```python
from build123d import *

# Parameters (mm, degrees)
BOSS_EXTRUDE1_DEPTH      = 60
BOSS_EXTRUDE1_DEPTH_BACK = 20
SKETCH2_R                = 1.7
CUT_EXTRUDE1_DEPTH       = 10
BOSS_EXTRUDE2_START      = 24
BOSS_EXTRUDE2_DEPTH      = 24
CUT_EXTRUDE2_START       = -10
SKETCH4_R                = 1.7
CUT_EXTRUDE2_DEPTH       = 10


with BuildPart() as part:
    # Sketch1 → Boss-Extrude1 (new, two sides: drawn at the far end of the back side and taken through both)
    with BuildSketch(Plane(origin=(190.645148, 0, 0), x_dir=(0, 0, -1), z_dir=(1, 0, 0)).offset(-BOSS_EXTRUDE1_DEPTH_BACK)):
        with BuildLine():
            Line((-240.970904961, 189.163538159), (-246.970904961, 189.163538159))
            Line((-246.970904961, 189.163538159), (-246.970904961, 173.663538158))
            Line((-246.970904961, 173.663538158), (-240.970904961, 173.663538158))
            Line((-240.970904961, 173.663538158), (-240.970904961, 179.413538158))
            Line((-240.970904961, 179.413538158), (-241.970904961, 179.413538158))
            ThreePointArc((-241.970904961, 179.413538158), (-243.970904961, 181.413538158), (-241.970904961, 183.413538158))
            Line((-241.970904961, 183.413538158), (-240.970904961, 183.413538158))
            Line((-240.970904961, 183.413538158), (-240.970904961, 189.163538159))
        make_face()
    extrude(amount=BOSS_EXTRUDE1_DEPTH + BOSS_EXTRUDE1_DEPTH_BACK)

    # Sketch2 → Cut-Extrude1 (cut)
    with BuildSketch(Plane.XY.offset(246.970904961)):
        with Locations((246.645148, 186.288538158)):
            Circle(SKETCH2_R)
        with Locations((222.645148, 186.288538158)):
            Circle(SKETCH2_R)
        with Locations((198.645148, 186.288538158)):
            Circle(SKETCH2_R)
        with Locations((174.645148, 186.288538158)):
            Circle(SKETCH2_R)
        with Locations((246.645148, 176.593153442)):
            Circle(SKETCH2_R)
        with Locations((222.645148, 176.593153442)):
            Circle(SKETCH2_R)
        with Locations((198.645148, 176.593153442)):
            Circle(SKETCH2_R)
        with Locations((174.645148, 176.593153442)):
            Circle(SKETCH2_R)
    extrude(amount=-CUT_EXTRUDE1_DEPTH, mode=Mode.SUBTRACT)

    # Sketch3 → Boss-Extrude2 (add)
    with BuildSketch(Plane.ZY.offset(-170.645148).offset(BOSS_EXTRUDE2_START)):
        with BuildLine():
            Line((241.970904961, 179.413538158), (240.970904961, 179.413538158))
            Line((240.970904961, 179.413538158), (240.970904961, 173.663538158))
            Line((240.970904961, 173.663538158), (246.970904961, 173.663538158))
            Line((246.970904961, 173.663538158), (246.970904961, 189.163538159))
            Line((246.970904961, 189.163538159), (240.970904961, 189.163538159))
            Line((240.970904961, 189.163538159), (240.970904961, 183.413538158))
            Line((240.970904961, 183.413538158), (241.970904961, 183.413538158))
            ThreePointArc((241.970904961, 183.413538158), (243.970904961, 181.413538158), (241.970904961, 179.413538158))
        make_face()
    extrude(amount=-BOSS_EXTRUDE2_DEPTH)

    # Sketch4 → Cut-Extrude2 (cut)
    with BuildSketch(Plane(origin=(0, 0, 240.970904961), x_dir=(-1, 0, 0), z_dir=(0, 0, -1)).offset(CUT_EXTRUDE2_START)):
        with Locations(Location((-174.645148, 176.593153442, 0), (0, 0, 180))):
            Circle(SKETCH4_R)
        with Locations(Location((-174.645148, 186.288538158, 0), (0, 0, 180))):
            Circle(SKETCH4_R)
        with Locations((-150.645148, 186.288538158)):
            Circle(SKETCH4_R)
        with Locations((-150.645148, 176.538538158)):
            Circle(SKETCH4_R)
    extrude(amount=CUT_EXTRUDE2_DEPTH, mode=Mode.SUBTRACT)


solid = part.part
```
Can you work these out from the model? Positions are in its coordinate system, mm. Round coordinates to 2 decimals unless told otherwise and drop trailing zeros. Order: outer loops, then holes, each group sorted by start corner. A loop starts at its lowest first (then second) coordinate and runs counter-clockwise, first axis right, second up. Notation, with made-up numbers: (26, -22) -> (84, -22) arc R16 cw to (84, 3) -> close; hole circle Ø7 at (83, 58). An arc over 180 degrees is marked (long way). Return JSON: item names as keys, results as strings. Group by question number.
1. If we section it at A-A, the plane z = 242.95: Count the separate pieces of the cut face and the enclosed holes in it, then the cut area to 3 significant figures.
2. If we section it at B-B, the plane x = 155.5: Write out the boundary of the cut face in (y, z), then the cut area to 3 significant figures.
3. Will these pins go through, and if not, where does the flat tip stop? pin 1 (3 mm diameter, centred on x = 246.65, y = 186.29, fed in from -Z); pin 2 (5.5 mm diameter, centred on x = 246.65, y = 176.59, fed in from -Z).
4. I need wall thicknesses on line 1 (X direction, y = 176.5, z = 244.8); line 2 (X direction, y = 186.5, z = 245.5); line 3 (Y direction, x = 218, z = 241.3). Which ranges of each line are inside material? Lowest first, please. Write a range as [from, to].
5. If we section it at C-C, the plane x = 198.5: Write out the boundary of the cut face in (y, z).
Output values:
{
 "1": {"separate pieces": "2", "enclosed holes": "10", "area": "1,160 mm²"},
 "2": {"outline": "(173.66, 240.97) -> (179.41, 240.97) -> (179.41, 241.97) arc R2 cw to (183.41, 241.97) -> (183.41, 240.97) -> (189.16, 240.97) -> (189.16, 246.97) -> (173.66, 246.97) -> close", "area": "82.7 mm²"},
 "3": {"pin 1": "through", "pin 2": "z = 240.97"},
 "4": {"line 1": "[146.65, 148.95], [152.34, 172.95], [176.34, 196.95], [200.34, 220.95], [224.34, 244.95], [248.34, 250.65]", "line 2": "[146.65, 148.96], [152.33, 172.96], [176.33, 196.96], [200.33, 220.96], [224.33, 244.96], [248.33, 250.65]", "line 3": "[173.66, 179.41], [183.41, 189.16]"},
 "5": {"outline": "(173.66, 240.97) -> (174.9, 240.97) -> (174.9, 246.97) -> (173.66, 246.97) -> close; (178.29, 240.97) -> (179.41, 240.97) -> (179.41, 241.97) arc R2 cw to (183.41, 241.97) -> (183.41, 240.97) -> (184.59, 240.97) -> (184.59, 246.97) -> (178.29, 246.97) -> close; (187.98, 240.97) -> (189.16, 240.97) -> (189.16, 246.97) -> (187.98, 246.97) -> close"}
}
